The model under review builds one solid part; all positions refer to its coordinate system, in mm. A direction names the side the tool comes from. Give positions to 0.01 mm unless a question says otherwise; leave off trailing zeros. Loops run counter-clockwise (first coordinate to the right, second up) from the corner with the lowest first, then second, coordinate; pieces in that order, holes last. Notation, with made-up numbers: (-14.5, 36) - (-6.5, 36) arc R33 ccw to (-6.5, 70) - close; hole circle Ø8 at (52, 12). An arc over 180 degrees is marked (long way). Answer as a JSON object with one key per item and string values.
from build123d import *

# Parameters (mm, degrees)
EXTRUDE_1_DEPTH     = 350
SKETCH_2_W          = 329
SKETCH_2_H          = 30
CUT_EXTRUDE_1_DEPTH = 470.574275275
SKETCH_3_R          = 5.15
CUT_EXTRUDE_2_DEPTH = 470.574275364


with BuildPart() as part:
    # 草图1 → 凸台-拉伸1 (new body)
    with BuildSketch(Plane.XY):
        with BuildLine():
            Line((-140, 0), (-140, -125))
            Line((-140, -125), (-130, -125))
            Line((-130, -125), (-130, 0))
            ThreePointArc((-130, 0), (0, 130), (130, 0))
            Line((130, 0), (130, -125))
            Line((130, -125), (140, -125))
            Line((140, -125), (140, 0))
            ThreePointArc((140, 0), (0, 140), (-140, 0))
        make_face()
    extrude(amount=EXTRUDE_1_DEPTH)

    # 草图2 → 切除-拉伸1 (cut, through all)
    with BuildSketch(Plane.ZY.offset(140)):
        with Locations((185.5, -110)):
            Rectangle(SKETCH_2_W, SKETCH_2_H)
        with BuildLine():
            Line((50, 140), (50, 0.249378106))
            ThreePointArc((50, 0.249378106), (62.927373322, -33.300887932), (95.024814049, -49.502481405))
            Line((95.024814049, -49.502481405), (350, -75))
            Line((350, -75), (350, 140))
            Line((350, 140), (50, 140))
        make_face()
    extrude(amount=-CUT_EXTRUDE_1_DEPTH, mode=Mode.SUBTRACT)

    # 草图3 → 切除-拉伸2 (cut, through all)
    with BuildSketch(Plane.ZY.offset(140)):
        with Locations(Location((120, -80, 0), (0, 0, 270))):
            Circle(SKETCH_3_R)
        with Locations(Location((250, -80, 0), (0, 0, 270))):
            Circle(SKETCH_3_R)
    extrude(amount=-CUT_EXTRUDE_2_DEPTH, mode=Mode.SUBTRACT)


solid = part.part
Q1. Consider section B-B, the plane y = -80. State the section outline as (x, z) points, plus the area to 3 significant figures.
Results:
{"outline": "(-140, 0) - (-130, 0) - (-130, 114.85) - (-140, 114.85) - close; (-140, 125.15) - (-130, 125.15) - (-130, 244.85) - (-140, 244.85) - close; (-140, 255.15) - (-130, 255.15) - (-130, 350) - (-140, 350) - close; (130, 0) - (140, 0) - (140, 114.85) - (130, 114.85) - close; (130, 125.15) - (140, 125.15) - (140, 244.85) - (130, 244.85) - close; (130, 255.15) - (140, 255.15) - (140, 350) - (130, 350) - close", "area": "6,590 mm^2"}
Q2. Consider section A-A, the plane z = 250. State the section outline as (x, y) points.
Results:
{"outline": "(-140, -95) - (-130, -95) - (-130, -85.15) - (-140, -85.15) - close; (-140, -74.85) - (-130, -74.85) - (-130, -65) - (-140, -65) - close; (130, -95) - (140, -95) - (140, -85.15) - (130, -85.15) - close; (130, -74.85) - (140, -74.85) - (140, -65) - (130, -65) - close"}
Q3. To check wall thickness, follow probe 1 along Z at (x, y) = (132.75, -80); probe 2 along X at (y, z) = (-80, 267.5); probe 3 along Y at (x, z) = (19.5, 20). State the ranges of each line that lie inside material, in increasing order. Write a range as [from, to].
Results:
{"probe 1": "z = [0, 114.85], [125.15, 244.85], [255.15, 350]", "probe 2": "x = [-140, -130], [130, 140]", "probe 3": "y = [128.53, 138.64]"}
Q4. For faces 1 (the face through (135, -85, 350)), 2 (the face through (-130, -77, 134)), 3 (the face through (135, -95, 183)), 4 (the face through (-1, 133, 50)), 5 (the face through (140, -77, 134)), list the 3-axis set-ups (+Z, -Z, +X, -X, +Y, -Y) from which the entire face can be reached by the end or side of a thin tool; tool diameter is ignored.
Results:
{"face 1": "+Z, +X, -X, +Y, -Y", "face 2": "+Z, -Z, -Y", "face 3": "+Z, +X, -X, -Y", "face 4": "+Z, +X, -X, +Y", "face 5": "+Z, -Z, +X, +Y, -Y"}
Q5. The part is to be moulded in two halves that separate along Y. For faces 6 (the face through (135, -125, 10)), 7 (the face through (134.93, -82.77, 254.34)), 8 (the face through (-135, -85, 350)), say which applies: +Y half, -Y half, draft (parallel to the pull), parting line (faces both ways), or undercut.
Results:
{"face 6": "-Y half", "face 7": "undercut", "face 8": "draft"}
Q6. Clearance check with flat-ended pins moving along their axes: pin 1 Ø8 at (x, y) = (-134.5, -112) entering from +Z; pin 2 Ø10 at (x, y) = (74, 107) entering from +Z; pin 3 Ø16.5 at (y, z) = (-80, 250) entering from +X; pin 4 Ø12 at (y, z) = (31, 55.5) entering from -X. State where each tip first meets the part, or that it passes through.
Results:
{"pin 1": "stops at z = 21", "pin 2": "stops at z = 50", "pin 3": "stops at x = 140", "pin 4": "stops at x = -137.05"}
Q7. Consider section C-C, the plane z = 140. State the section outline as (x, y) points.
Results:
{"outline": "(-140, -95) - (-130, -95) - (-130, -54) - (-140, -54) - close; (130, -95) - (140, -95) - (140, -54) - (130, -54) - close"}
Q8. Consider section D-D, the plane y = 95. State the section outline as (x, z) points, plus the area to 3 significant figures.
Results:
{"outline": "(-102.83, 0) - (-88.74, 0) - (-88.74, 50) - (-102.83, 50) - close; (88.74, 0) - (102.83, 0) - (102.83, 50) - (88.74, 50) - close", "area": "1,410 mm^2"}
